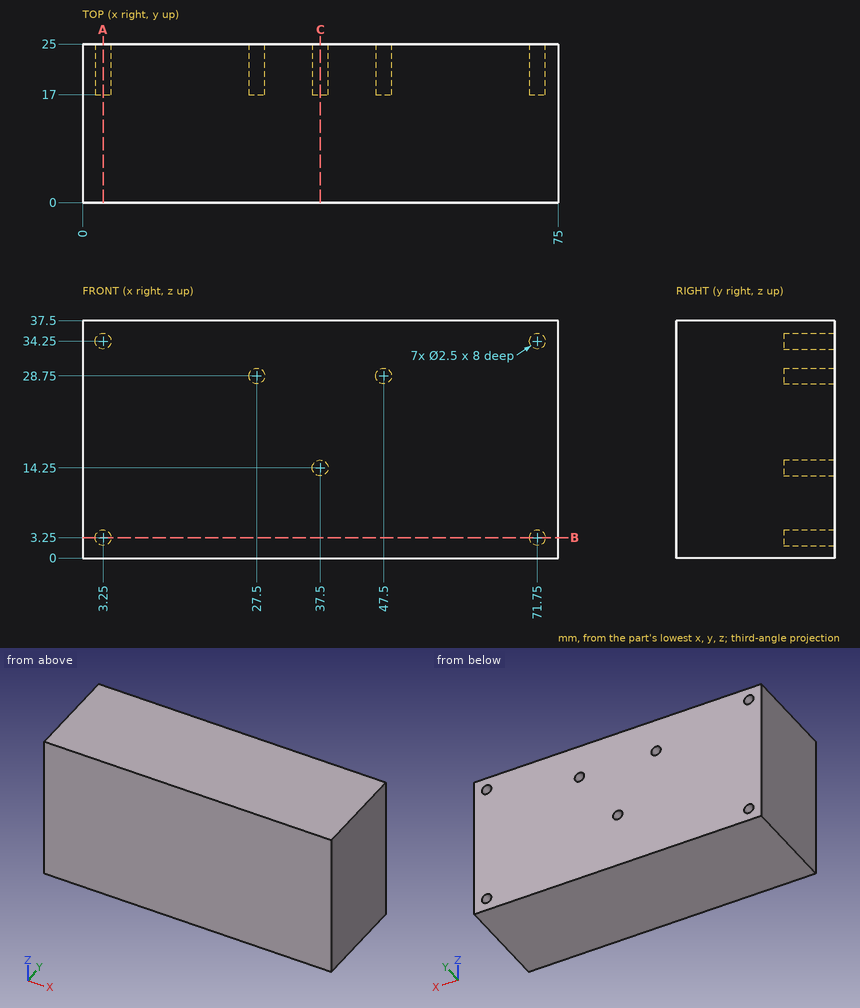
Study the drawing (mm; zero at the part's minimum x, y, z) and answer. Give positions to 0.01 mm unless a question says otherwise; leave off trailing zeros. Loops run counter-clockwise (first coordinate to the right, second up) from the corner with the lowest first, then second, coordinate; pieces in that order, holes last. Notation, with made-up numbers: (34, 75) - (62, 75) arc R8 ccw to (62, 80) - close; hole circle Ø9 at (69.5, -13). An arc over 180 degrees is marked (long way). Answer in a Markdown table with one row per item. Add a question column.
Q1. Consider line 1 along Z through (x, y) = (71.75, 19.25); line 2 along Z through (x, y) = (37.5, 21.5). Determine where each line is inside the solid, lowest interval first.
Q2. Each of these flat-tipped pins is pushed along its axis until it touches: P1, Ø2, axis at x = 27.5, z = 28.75, coming from the -Y side; P2, Ø1.5, axis at x = 37.5, z = 14.25, coming from the +Y side. Where does it stop, or does it pass through?
Q3. The part is cut by section C-C (x = 37.5). Determine the outline of the cut face in (y, z).
Q4. The part is cut by section A-A (x = 3.25). Determine the outline of the cut face in (y, z).
Q5. The part is cut by section B-B (z = 3.25). Determine the outline of the cut face in (x, y), and give its area (4 significant figures).
Solution:
| question | item | result |
|---|---|---|
| 1 | line 1 | z = 0 to 2, 4.5 to 33, 35.5 to 37.5 |
| 1 | line 2 | z = 0 to 13, 15.5 to 37.5 |
| 2 | P1 | stops at y = 0 |
| 2 | P2 | stops at y = 17 |
| 3 | outline | (0, 0) - (25, 0) - (25, 13) - (17, 13) - (17, 15.5) - (25, 15.5) - (25, 37.5) - (0, 37.5) - close |
| 4 | outline | (0, 0) - (25, 0) - (25, 2) - (17, 2) - (17, 4.5) - (25, 4.5) - (25, 33) - (17, 33) - (17, 35.5) - (25, 35.5) - (25, 37.5) - (0, 37.5) - close |
| 5 | outline | (0, 0) - (75, 0) - (75, 25) - (73, 25) - (73, 17) - (70.5, 17) - (70.5, 25) - (4.5, 25) - (4.5, 17) - (2, 17) - (2, 25) - (0, 25) - close |
| 5 | area | 1,835 mm² |
